```python
from build123d import *

# Parameters (mm, degrees)
F0_W     = 465
F0_H     = 117
F1_DEPTH = 50
F2_T     = -2
F4_R     = 7
F3_W     = 180
F3_H     = 60
F3_W_2   = 20
F3_H_2   = 20
F3_W_3   = 93
F3_H_3   = 36
F3_R     = 1.5
F3_W_4   = 77
F3_H_4   = 77
F3_R_2   = 9.5
F3_R_3   = 35
F5_DEPTH = 25
F6_R     = 5


with BuildPart() as f1:
    # F0 (on Front) → F1 (new body)
    with BuildSketch(Plane.XZ):
        with Locations((-12.6529467106, 27.1878533959)):
            Rectangle(F0_W, F0_H)
    extrude(amount=F1_DEPTH)

    # F2
    f2_openings = [f1.faces().sort_by_distance(p)[0] for p in [
        (-12.652947, 0, 27.187853),
    ]]
    offset(amount=F2_T, openings=f2_openings)

    # F4
    f4_edges = [f1.edges().sort_by_distance(p)[0] for p in [
        (-245.152947, -25, 85.687853),
        (219.847053, -25, 85.687853),
        (219.847053, -25, -31.312147),
        (-245.152947, -25, -31.312147),
        (-243.152947, -24, 83.687853),
        (-243.152947, -24, -29.312147),
        (217.847053, -24, -29.312147),
        (217.847053, -24, 83.687853),
    ]]
    fillet(f4_edges, radius=F4_R)

    # F3 (on face) → F5 (cut)
    with BuildSketch(Plane.XZ.offset(50)):
        with Locations((-49.312419115, 48.5197262004)):
            Rectangle(F3_W, F3_H)
        with Locations((76.3836680665, 68.3190373614)):
            Rectangle(F3_W_2, F3_H_2)
        Polygon((194.7213235501, 76.111191912), (114.5203134233, 76.111191912), (104.6208184867, 66.2116969754), (104.6208184867, -13.9893131514), (114.5203134233, -23.888808088), (194.7213235501, -23.888808088), (204.6208184867, -13.9893131514), (204.6208184867, 66.2116969754), align=None)
        with Locations((-81.5471372292, -73.4631650165)):
            Rectangle(F3_W_3, F3_H_3)
        with Locations((46.5855184052, 67.5480939005)):
            Circle(F3_R)
        with Locations((46.5855184052, 47.158148972)):
            Circle(F3_R)
        with Locations((46.5855184052, 26.052269754)):
            Circle(F3_R)
        with Locations((-195.3124095783, -98.1716645822)):
            Rectangle(F3_W_4, F3_H_4)
        with Locations((107.5167332374, 72.8625404379)):
            Circle(F3_R)
        with Locations((80.878779198, -82.3583360478)):
            Rectangle(F3_W_3, F3_H_3)
        with Locations((51.3206828289, -84.0745766136)):
            Circle(F3_R_2, mode=Mode.SUBTRACT)
        with Locations((81.3476530956, -84.0745766136)):
            Circle(F3_R_2, mode=Mode.SUBTRACT)
        with Locations((123.378779198, -96.3583360478)):
            Circle(F3_R, mode=Mode.SUBTRACT)
        with Locations((110.7360261029, -84.0745766136)):
            Circle(F3_R_2, mode=Mode.SUBTRACT)
        with Locations((38.378779198, -68.3583360478)):
            Circle(F3_R, mode=Mode.SUBTRACT)
        Polygon((-66.2842570873, 3.6055132091), (-130.7279079012, 3.6055132091), (-138.5060824942, -4.172661384), (-138.5060824942, -17.6163121979), (-130.7279079012, -25.3944867909), (-66.2842570873, -25.3944867909), (-58.5060824942, -17.6163121979), (-58.5060824942, -4.172661384), align=None)
        with Locations((-136.0060824942, 1.1055132091)):
            Circle(F3_R)
        with Locations((-136.0060824942, -22.8944867909)):
            Circle(F3_R)
        with Locations((-61.0060824942, 1.1055132091)):
            Circle(F3_R)
        with Locations((-61.0060824942, -22.8944867909)):
            Circle(F3_R)
        with Locations((107.5167332374, -20.8455865502)):
            Circle(F3_R)
        with Locations((202.0370356229, -20.8455660029)):
            Circle(F3_R)
        with Locations((202.0370356229, 72.8625404379)):
            Circle(F3_R)
        with Locations((-195.4793932134, 12.7347313118)):
            Circle(F3_R_3)
        with Locations((-144.8539147958, 67.5480939005)):
            Circle(F3_R)
        with Locations((-144.8539147958, 47.158148972)):
            Circle(F3_R)
        with Locations((-144.8539147958, 26.052269754)):
            Circle(F3_R)
        with Locations((-227.2830040105, 46.6578847659)):
            Circle(F3_R)
        with Locations((-227.2830040105, -19.1012599602)):
            Circle(F3_R)
        with Locations((-163.6415483004, -19.1012599602)):
            Circle(F3_R)
        with Locations((-5.8271809206, -7.7349814937)):
            Rectangle(F3_W_3, F3_H_3)
        with Locations((-163.6757824164, 46.6578847659)):
            Circle(F3_R)
    extrude(amount=-F5_DEPTH, mode=Mode.SUBTRACT)

    # F6
    f6_edges = [f1.edges().sort_by_distance(p)[0] for p in [
        (217.796801, -50, 83.637601),
    ]]
    fillet(f6_edges, radius=F6_R)


solid = f1.part
```
CAD build for the part. Positions are in the model's coordinates, mm. A direction names the side the tool comes from. Round coordinates to 2 decimals unless told otherwise and drop trailing zeros. Order: outer loops, then holes, each group sorted by start corner. A loop starts at its lowest first (then second) coordinate and runs counter-clockwise, first axis right, second up. Notation, with made-up numbers: (78.5, 15) - (88.5, 15) arc R7 cw to (88.5, 20) - close; hole circle Ø8 at (58, 85). An arc over 180 degrees is marked (long way). Answer in a Markdown table with one row per item. Add a question column.
(1) Band-saw the part on B-B on y = -29. List the corners of the cut face in (x, z), and give its area (3 significant figures).
(2) Band-saw the part on A-A on x = 36.5. List the corners of the cut face in (y, z), and give its area (3 significant figures).
(3) Band-saw the part on C-C on z = 39. List the corners of the cut face in (x, y), and give its area (3 significant figures).
(4) Band-saw the part on D-D on x = -212.5. List the corners of the cut face in (y, z).
(5) Drop flat-ended pins along their axis: pin 1 Ø3.5 at (x, z) = (-61.01, -22.89) entering from +Y; pin 2 Ø1.6 at (x, y) = (-83, -49) entering from +Z; pin 3 Ø1 at (x, y) = (-10.5, -48.5) entering from -Z. Give the stop position or say it passes through.
(6) Probe L1, parallel to Z at x = -182, y = -3.5; L2, parallel to X at y = -33, z = -5.5; L3, parallel to Y at x = 56.5, z = 19.5. List the from-to ranges inside material, lowest first. Write a range as [from, to].
(7) Mould opens along X. For faces 4 (the face through (-16, -22, -31.312)), 5 (the face through (219.847, -22, 26)), 6 (the face through (-134.67, -49.01, -21.45)) say: +X half, -X half, draft (parallel to the pull), parting line (faces both ways), or undercut.
(8) 3-axis set-ups, long thin cutter, end or side, ignore diameter. For faces 1 (the face through (-245.153, -22, 26)), 2 (the face through (-243.153, -24, 26)), 3 (the face through (-62.34, -49.01, -0.34)): which of +Z, -Z, +X, -X, +Y, -Y reach the whole face in a straight line?
Data:
| question | item | result |
|---|---|---|
| 1 | outline | (-245.15, -24.31) arc R7 ccw to (-238.15, -31.31) - (212.85, -31.31) arc R7 ccw to (219.85, -24.31) - (219.85, 78.69) arc R7 ccw to (212.85, 85.69) - (-238.15, 85.69) arc R7 ccw to (-245.15, 78.69) - close; hole (-243.15, -22.31) arc R7 ccw to (-236.15, -29.31) - (210.85, -29.31) arc R7 ccw to (217.85, -22.31) - (217.85, 76.69) arc R7 ccw to (210.85, 83.69) - (-236.15, 83.69) arc R7 ccw to (-243.15, 76.69) - close |
| 1 | area | 2,310 mm^2 |
| 2 | outline | (-50, -26.31) arc R5 ccw to (-45, -31.31) - (0, -31.31) - (0, -29.31) - (-48, -29.31) - (-48, -25.73) - (-50, -25.73) - close; (-50, 10.27) - (-48, 10.27) - (-48, 18.52) - (-50, 18.52) - close; (-50, 78.52) - (-48, 78.52) - (-48, 83.69) - (0, 83.69) - (0, 85.69) - (-45, 85.69) arc R5 ccw to (-50, 80.69) - close |
| 2 | area | 223 mm^2 |
| 3 | outline | (-245.15, -45) arc R5 ccw to (-240.15, -50) - (-218.61, -50) - (-218.61, -48) - (-243.15, -48) - (-243.15, 0) - (-245.15, 0) - close; (-172.35, -50) - (-139.31, -50) - (-139.31, -48) - (-172.35, -48) - close; (40.69, -50) - (104.62, -50) - (104.62, -48) - (40.69, -48) - close; (204.62, -50) - (214.85, -50) arc R5 ccw to (219.85, -45) - (219.85, 0) - (217.85, 0) - (217.85, -48) - (204.62, -48) - close |
| 3 | area | 459 mm^2 |
| 4 | outline | (-50, -26.31) arc R5 ccw to (-45, -31.31) - (0, -31.31) - (0, -29.31) - (-48, -29.31) - (-48, -17.85) - (-50, -17.85) - close; (-50, 43.32) - (-48, 43.32) - (-48, 83.69) - (0, 83.69) - (0, 85.69) - (-45, 85.69) arc R5 ccw to (-50, 80.69) - close |
| 5 | pin 1 | stops at y = -48 |
| 5 | pin 2 | stops at z = 84.53 |
| 5 | pin 3 | stops at z = -30.31 |
| 6 | L1 | z = [-31.31, -29.31], [83.69, 85.69] |
| 6 | L2 | x = [-245.15, -243.15], [217.85, 219.85] |
| 6 | L3 | y = [-50, -48] |
| 7 | face 4 | draft |
| 7 | face 5 | +X half |
| 7 | face 6 | undercut |
| 8 | face 1 | +Z, -Z, -X, +Y, -Y |
| 8 | face 2 | +Y |
| 8 | face 3 | +Y, -Y |
